```python
from build123d import *

# Parameters (mm, degrees)
PAD_DEPTH            = 62
PAD001_DEPTH         = 62
FILLET_R             = 4.5
SKETCH001_R          = 6.35
SKETCH001_R_2        = 2.5
POCKET_DEPTH         = 50.801
LINEARPATTERN_COUNT  = 2
LINEARPATTERN_PITCH  = 80
SKETCH002_R          = 5.357812
SKETCH002_R_2        = 2.5
POCKET001_DEPTH      = 50.801
POCKET001_DEPTH_BACK = 0.001
SKETCH003_W          = 60
SKETCH003_H          = 51.1187
POCKET002_DEPTH      = 286.617678
POCKET002_DEPTH_BACK = 337.417678
SKETCH004_R          = 1.865
SKETCH004_R_2        = 0.05
POCKET003_DEPTH      = 0.001
POCKET003_DEPTH_BACK = 50.801
SKETCH005_W          = 60
SKETCH005_H          = 12.25
POCKET004_DEPTH      = 62.001
POCKET004_DEPTH_BACK = 62.001
SKETCH006_W          = 37.3666
SKETCH006_H          = 44.7638
POCKET005_DEPTH      = 286.617678
POCKET005_DEPTH_BACK = 337.417678
SKETCH007_R          = 2.5
POCKET006_DEPTH      = 286.617678
POCKET006_DEPTH_BACK = 337.417678
SKETCH008_R          = 1.25
HOLE_DEPTH           = 10
HOLE_TIPS_R          = 1.25


with BuildPart() as part:
    # Sketch → Pad (new body)
    with BuildSketch(Plane.XY):
        Polygon((0, 0), (50.8, 0), (50.8, -6.35), (6.35, -6.35), (6.35, -50.8), (0, -50.8), align=None)
    extrude(amount=-PAD_DEPTH)

    # Sketch → Pad001 (join)
    with BuildSketch(Plane.XY):
        Polygon((0, 0), (50.8, 0), (50.8, -6.35), (6.35, -6.35), (6.35, -50.8), (0, -50.8), align=None)
    extrude(amount=PAD001_DEPTH)

    # Fillet
    fillet_edges = [part.edges().sort_by_distance(p)[0] for p in [
        (6.35, -50.8, 0),
        (6.35, -6.35, 0),
        (50.8, -6.35, 0),
    ]]
    fillet(fillet_edges, radius=FILLET_R)

    # Sketch001 → Pocket (cut, through all)
    with BuildSketch(Plane.YZ):
        with Locations((-14, -40)):
            Circle(SKETCH001_R)
        with Locations((-14, -24)):
            Circle(SKETCH001_R_2)
        with Locations((-14, -56)):
            Circle(SKETCH001_R_2)
    pocket = extrude(amount=POCKET_DEPTH, mode=Mode.SUBTRACT)

    # LinearPattern: Pocket ×2
    with Locations(*[(0, 0, i * LINEARPATTERN_PITCH) for i in range(1, LINEARPATTERN_COUNT)]):
        add(pocket, mode=Mode.SUBTRACT)

    # Sketch002 → Pocket001 (cut, two sides)
    with BuildSketch(Plane.YZ) as pocket001_sk:
        with Locations((-39, 0)):
            Circle(SKETCH002_R)
        with Locations((-39, 18)):
            Circle(SKETCH002_R_2)
        with Locations((-39, -18)):
            Circle(SKETCH002_R_2)
    extrude(amount=POCKET001_DEPTH, mode=Mode.SUBTRACT)
    extrude(pocket001_sk.sketch, amount=-POCKET001_DEPTH_BACK, mode=Mode.SUBTRACT)

    # Sketch003 → Pocket002 (cut, two sides)
    with BuildSketch(Plane.XZ) as pocket002_sk:
        with Locations((36.35, 225.55935)):
            Rectangle(SKETCH003_W, SKETCH003_H)
    pocket002 = extrude(amount=-POCKET002_DEPTH, mode=Mode.SUBTRACT) + extrude(pocket002_sk.sketch, amount=POCKET002_DEPTH_BACK, mode=Mode.SUBTRACT)

    # Mirrored001: Pocket002 across Sketch003 H_Axis
    add(pocket002.mirror(Plane(origin=(0, 0, 0), x_dir=(0, -1, 0), z_dir=(0, 0, 1))), mode=Mode.SUBTRACT)

    # Sketch004 → Pocket003 (cut, two sides)
    with BuildSketch(Plane.XZ) as pocket003_sk:
        with Locations((45, 15)):
            Circle(SKETCH004_R)
        with Locations((45, -15)):
            Circle(SKETCH004_R)
        with Locations((23, 15)):
            Circle(SKETCH004_R)
        with Locations((23, -15)):
            Circle(SKETCH004_R)
        with Locations((34, 0)):
            Circle(SKETCH004_R_2)
    extrude(amount=-POCKET003_DEPTH, mode=Mode.SUBTRACT)
    extrude(pocket003_sk.sketch, amount=POCKET003_DEPTH_BACK, mode=Mode.SUBTRACT)

    # Sketch005 → Pocket004 (cut, two sides)
    with BuildSketch(Plane.XY) as pocket004_sk:
        with Locations((36.35, -12.125)):
            Rectangle(SKETCH005_W, SKETCH005_H)
    extrude(amount=-POCKET004_DEPTH, mode=Mode.SUBTRACT)
    extrude(pocket004_sk.sketch, amount=POCKET004_DEPTH_BACK, mode=Mode.SUBTRACT)

    # Sketch006 → Pocket005 (cut, two sides)
    with BuildSketch(Plane.YZ) as pocket005_sk:
        with Locations((-43.4833, 47.3819)):
            Rectangle(SKETCH006_W, SKETCH006_H)
    pocket005 = extrude(amount=-POCKET005_DEPTH, mode=Mode.SUBTRACT) + extrude(pocket005_sk.sketch, amount=POCKET005_DEPTH_BACK, mode=Mode.SUBTRACT)

    # Mirrored: Pocket005 across Sketch006 H_Axis
    add(pocket005.mirror(Plane.XY), mode=Mode.SUBTRACT)

    # Sketch007 → Pocket006 (cut, two sides)
    with BuildSketch(Plane.XZ) as pocket006_sk:
        with Locations((23, 54)):
            Circle(SKETCH007_R)
        with Locations((47, 54)):
            Circle(SKETCH007_R)
        with Locations((47, 36)):
            Circle(SKETCH007_R)
        with Locations((23, 36)):
            Circle(SKETCH007_R)
    pocket006 = extrude(amount=-POCKET006_DEPTH, mode=Mode.SUBTRACT) + extrude(pocket006_sk.sketch, amount=POCKET006_DEPTH_BACK, mode=Mode.SUBTRACT)

    # Mirrored002: Pocket006 across Sketch007 H_Axis
    add(pocket006.mirror(Plane(origin=(0, 0, 0), x_dir=(0, -1, 0), z_dir=(0, 0, 1))), mode=Mode.SUBTRACT)

    # Sketch008 (on Face3 of Mirrored002) → Hole (cut)
    with BuildSketch(Plane(origin=(0, 0, 0), x_dir=(-1, 0, 0), z_dir=(0, 1, 0))):
        with Locations((-18, -7.5)):
            Circle(SKETCH008_R)
        with Locations((-3, -7.5)):
            Circle(SKETCH008_R)
        with Locations((-3, -22.5)):
            Circle(SKETCH008_R)
        with Locations((-18, -22.5)):
            Circle(SKETCH008_R)
        with Locations((-3, 7.5)):
            Circle(SKETCH008_R)
        with Locations((-3, 22.5)):
            Circle(SKETCH008_R)
        with Locations((-18, 22.5)):
            Circle(SKETCH008_R)
        with Locations((-18, 7.5)):
            Circle(SKETCH008_R)
    extrude(amount=-HOLE_DEPTH, mode=Mode.SUBTRACT)

    # Hole tips → Hole tip 1 section 0
    with BuildSketch(Plane(origin=(0, -10, 0), x_dir=(-1, 0, 0), z_dir=(0, 1, 0)), mode=Mode.PRIVATE) as hole_tip_1_s0:
        with Locations((-18, -7.5)):
            Circle(HOLE_TIPS_R)
    loft([hole_tip_1_s0.sketch, Vertex(18, -10.751076, -7.5)], mode=Mode.SUBTRACT)

    # Hole tips → Hole tip 2 section 0
    with BuildSketch(Plane(origin=(0, -10, 0), x_dir=(-1, 0, 0), z_dir=(0, 1, 0)), mode=Mode.PRIVATE) as hole_tip_2_s0:
        with Locations((-3, -7.5)):
            Circle(HOLE_TIPS_R)
    loft([hole_tip_2_s0.sketch, Vertex(3, -10.751076, -7.5)], mode=Mode.SUBTRACT)

    # Hole tips → Hole tip 3 section 0
    with BuildSketch(Plane(origin=(0, -10, 0), x_dir=(-1, 0, 0), z_dir=(0, 1, 0)), mode=Mode.PRIVATE) as hole_tip_3_s0:
        with Locations((-3, -22.5)):
            Circle(HOLE_TIPS_R)
    loft([hole_tip_3_s0.sketch, Vertex(3, -10.751076, -22.5)], mode=Mode.SUBTRACT)

    # Hole tips → Hole tip 4 section 0
    with BuildSketch(Plane(origin=(0, -10, 0), x_dir=(-1, 0, 0), z_dir=(0, 1, 0)), mode=Mode.PRIVATE) as hole_tip_4_s0:
        with Locations((-18, -22.5)):
            Circle(HOLE_TIPS_R)
    loft([hole_tip_4_s0.sketch, Vertex(18, -10.751076, -22.5)], mode=Mode.SUBTRACT)

    # Hole tips → Hole tip 5 section 0
    with BuildSketch(Plane(origin=(0, -10, 0), x_dir=(-1, 0, 0), z_dir=(0, 1, 0)), mode=Mode.PRIVATE) as hole_tip_5_s0:
        with Locations((-3, 7.5)):
            Circle(HOLE_TIPS_R)
    loft([hole_tip_5_s0.sketch, Vertex(3, -10.751076, 7.5)], mode=Mode.SUBTRACT)

    # Hole tips → Hole tip 6 section 0
    with BuildSketch(Plane(origin=(0, -10, 0), x_dir=(-1, 0, 0), z_dir=(0, 1, 0)), mode=Mode.PRIVATE) as hole_tip_6_s0:
        with Locations((-3, 22.5)):
            Circle(HOLE_TIPS_R)
    loft([hole_tip_6_s0.sketch, Vertex(3, -10.751076, 22.5)], mode=Mode.SUBTRACT)

    # Hole tips → Hole tip 7 section 0
    with BuildSketch(Plane(origin=(0, -10, 0), x_dir=(-1, 0, 0), z_dir=(0, 1, 0)), mode=Mode.PRIVATE) as hole_tip_7_s0:
        with Locations((-18, 22.5)):
            Circle(HOLE_TIPS_R)
    loft([hole_tip_7_s0.sketch, Vertex(18, -10.751076, 22.5)], mode=Mode.SUBTRACT)

    # Hole tips → Hole tip 8 section 0
    with BuildSketch(Plane(origin=(0, -10, 0), x_dir=(-1, 0, 0), z_dir=(0, 1, 0)), mode=Mode.PRIVATE) as hole_tip_8_s0:
        with Locations((-18, 7.5)):
            Circle(HOLE_TIPS_R)
    loft([hole_tip_8_s0.sketch, Vertex(18, -10.751076, 7.5)], mode=Mode.SUBTRACT)


solid = part.part
```
The listing builds one solid part. Answer for the finished solid, in the listing's coordinates (mm). A direction names the side the tool comes from. Give positions to 0.01 mm unless a question says otherwise; leave off trailing zeros. Write each loop counter-clockwise with the first axis right and the second up, starting at its lowest first coordinate (ties: lowest second). Pieces come first, ordered by that corner, then holes. Notation, with made-up numbers: (28.25, 67.25) -> (83.25, 67.25) arc R20 cw to (83.25, 104.25) -> close; hole circle Ø9 at (57, 12). An arc over 180 degrees is marked (long way). Write item = value, one per line. Start each with the question number.
1) Each of these flat-tipped pins is pushed along its axis until it touches: pin 1 (3 mm diameter, centred on x = 23, z = -15, fed in from -Y); pin 2 (1.5 mm diameter, centred on x = 3, z = -22.5, fed in from -Y); pin 3 (4.5 mm diameter, centred on x = 23, z = 15, fed in from -Y); pin 4 (2 mm diameter, centred on x = 3, z = 22.5, fed in from +Y). Where does it stop, or does it pass through?
2) Determine the mould class of faces 4 (the face through (50.03, -4.37, -0.87)), 5 (the face through (0, -20, -1)), 6 (the face through (3.1, -16.5, 56.1)), 7 (the face through (16.845, -2.958, -7.979)) for opening direction X: +X half, -X half, draft (parallel to the pull), parting line (faces both ways), or undercut.
3) Straight lines are drawn through the part: line 1 along Z through (x, y) = (3, -5); line 2 along Z through (x, y) = (1, -39); line 3 along X through (y, z) = (-4, -7). For each, find the intervals that lie inside material, in ascending order.
4) The part is cut by section D-D, the plane x = 36. Determine the outline of the cut face in (y, z).
5) Which of the six approach directions +Z, -Z, +X, -X, +Y, -Y give full straight-line access (tool end or side, diameter ignored) to faces 1 (the face through (3, -38, -25)), 2 (the face through (22.46, -2.96, 33.56)), 3 (the face through (3, -38, 25))?
6) The part is cut by section B-B, the plane z = -36. Determine the outline of the cut face in (x, y), and give its area (3 significant figures).
7) The part is cut by section A-A, the plane y = -14. Determine the outline of the cut face in (x, z), and give its area (3 significant figures).
8) The part is cut by section C-C, the plane y = -31. Determine the outline of the cut face in (x, z).
Solutions:
q1.pin_1 = through
q1.pin_2 = -50.78
q1.pin_3 = -6
q1.pin_4 = -10.15
q2.face_4 = +X half
q2.face_5 = -X half
q2.face_6 = draft
q2.face_7 = undercut
q3.line_1 = -62 to -23.75, -21.25 to -8.75, -6.25 to 6.25, 8.75 to 21.25, 23.75 to 62
q3.line_2 = -25 to -20.5, -15.5 to -5.36, 5.36 to 15.5, 20.5 to 25
q3.line_3 = 0 to 1.85, 4.15 to 16.85, 19.15 to 50.25
q4.outline = (-6, -62) -> (0, -62) -> (0, 62) -> (-6, 62) -> close
q5.face_1 = -Z, +X, -X, -Y
q5.face_2 = +Y, -Y
q5.face_3 = +Z, +X, -X, -Y
q6.outline = (0, -24.8) -> (6.35, -24.8) -> (6.35, -18.93) -> (0, -18.93) -> close; (0, -9.07) -> (6.35, -9.07) -> (6.35, -6) -> (20.5, -6) -> (20.5, 0) -> (0, 0) -> close; (25.5, -6) -> (44.5, -6) -> (44.5, 0) -> (25.5, 0) -> close; (49.5, -5.01) arc R4.5 ccw to (50.8, -1.85) -> (50.8, 0) -> (49.5, 0) -> close
q6.area = 299 mm²
q7.outline = (0, -62) -> (6.35, -62) -> (6.35, -58.5) -> (0, -58.5) -> close; (0, -53.5) -> (6.35, -53.5) -> (6.35, -46.35) -> (0, -46.35) -> close; (0, -33.65) -> (6.35, -33.65) -> (6.35, -26.5) -> (0, -26.5) -> close; (0, -21.5) -> (6.35, -21.5) -> (6.35, 21.5) -> (0, 21.5) -> close; (0, 26.5) -> (6.35, 26.5) -> (6.35, 33.65) -> (0, 33.65) -> close; (0, 46.35) -> (6.35, 46.35) -> (6.35, 53.5) -> (0, 53.5) -> close; (0, 58.5) -> (6.35, 58.5) -> (6.35, 62) -> (0, 62) -> close
q7.area = 499 mm²
q8.outline = (0, -25) -> (6.35, -25) -> (6.35, 25) -> (0, 25) -> close
